The model under review builds one solid part; all positions refer to its coordinate system, in mm. Coordinates: 2 decimals unless noted, no trailing zeros. Loops run counter-clockwise (first coordinate to the right, second up) from the corner with the lowest first, then second, coordinate; pieces in that order, holes last. Notation, with made-up numbers: M 11,73.5 L 39,73.5 A21 ccw 39,92.5 Z; hole C -32,78 d6. An arc over 180 degrees is marked long. Write item = value, one per line. Start each with the question number.
Q1. We need section C-C on y = 118.25. Give the boundary of the cut face in (x, z) (1 decimal), and give its area (3 significant figures).
Q2. We need section A-A on z = -185.5. Give the boundary of the cut face in (x, y), and give its area (3 significant figures).
Q3. Wall thickness on probe 1 along Z at (x, y) = (-131, 114.5) (3 decimals); probe 2 along X at (y, z) = (118.75, -142); probe 3 along X at (y, z) = (114.5, -168): over which ranges is each line inside the solid? List them lowest first.
Q4. We need section B-B on x = -75. Give the boundary of the cut face in (y, z) (3 decimals).
Q5. Mouldability with a two-part tool opening along Z and no side actions: class faces 1 (the face through (-130.53, 116.83, -199.47)), 2 (the face through (-91, 117, -250.645)), 3 (the face through (-91, 117, -75.645)) as released by +Z, released by -Z, zero draft, split by the parting line, or undercut.
Autodesk Inventor part; units mm, degrees
ref_plane "YZ Plane" through (0, 0, 0) normal (1, 0, 0) x (0, 1, 0)
ref_plane "XZ Plane" through (0, 0, 0) normal (0, 1, 0) x (-1, 0, 0)
ref_plane "XY Plane" through (0, 0, 0) normal (0, 0, 1) x (1, 0, 0)
ref_plane "Work Plane2" through (-92.9211, 111.7581, -85.645) normal (0, 1, 0) x (-1, 0, 0)
sketch "Sketch2" plane through (-92.9211, 111.7581, -85.645) normal (0, 1, 0) x (-1, 0, 0)
  line L0 (63, 0) -> (-63, 0)
  line L1 (-63, 0) -> (-63, -150)
  line L2 (-63, -150) -> (63, -150)
  line L3 (63, -150) -> (63, 0)
  line L4 (63, 0) -> (-63, -150) construction
  line L5 (-63, 0) -> (63, -150) construction
  line L6 (-114.9576, 160) -> (114.9576, 160)
  line L7 (114.9576, 160) -> (114.9576, -160)
  line L8 (114.9576, -160) -> (-114.9576, -160)
  line L9 (-114.9576, -160) -> (-114.9576, 160)
  line L10 (119.9576, -165) -> (119.9576, 165)
  line L11 (119.9576, 165) -> (-119.9576, 165)
  line L12 (-119.9576, 165) -> (-119.9576, 10)
  line L13 (-119.9576, -165) -> (119.9576, -165)
  line L14 (-119.9576, 10) -> (-114.9576, 10)
  line L15 (-114.9576, 10) -> (114.9576, 10)
  line L16 (114.9576, 10) -> (119.9576, 10)
  line L17 (-119.9576, 10) -> (-119.9576, -165)
  point P0 (-92.9211, 85.645)
  point P1 (0, -75)
  point P2 (114.9576, 160)
  dimension "d0" = 126
  dimension "d1" = 150
  dimension "d2" = 5
  dimension "d5" = 10
  dimension "d6" = 10
extrude "Extrusion1" add sketch "Sketch2" along normal blind 10 contours L3 L2 L1 L0 | L15 L7 L8 L9 | L9 L8 L7 L16 L10 L13 L17 L14
sketch "Sketch3" plane through (-92.9211, 111.7581, -85.645) normal (0, -1, 0) x (1, 0, 0)
  line L0 (-119.9576, 10) -> (119.9576, 10)
  line L1 (-119.9576, -165) -> (-119.9576, 10)
  line L2 (119.9576, -165) -> (-119.9576, -165)
  line L3 (119.9576, 10) -> (119.9576, -165)
  line L4 (-119.9576, -165) -> (119.9576, 10)
  line L5 (-119.9576, 10) -> (119.9576, -165)
  circle A0 centre (0, -77.5) radius 37.5
  point P0 (92.9211, 85.645)
  dimension "d7" = 75
extrude "Extrusion2" cut sketch "Sketch3" against normal through all contours A0 L4 L5 | L5 L4 A0 | A0 L5 L4 | L4 L5 A0
sketch "Sketch4" plane through (-92.9211, 111.7581, -85.645) normal (0, -1, 0) x (1, 0, 0)
  circle A0 centre (-37.5, -38.6758) radius 2.5
  circle A1 centre (37.5, -38.6758) radius 2.5
  circle A2 centre (37.5, -116.3242) radius 2.5
  circle A3 centre (-37.5, -116.3242) radius 2.5
  arc A4 (47.5, -35) -> (42.5, -30) centre (42.5, -35) ccw
  line L0 (42.5, -30) -> (-42.5, -30)
  arc A5 (-42.5, -30) -> (-47.5, -35) centre (-42.5, -35) ccw
  line L1 (-47.5, -35) -> (-47.5, -120)
  arc A6 (-47.5, -120) -> (-42.5, -125) centre (-42.5, -120) ccw
  line L2 (-42.5, -125) -> (42.5, -125)
  arc A7 (42.5, -125) -> (47.5, -120) centre (42.5, -120) ccw
  line L3 (47.5, -120) -> (47.5, -35)
  circle A8 centre (0, -77.5) radius 5
  point P0 (92.9211, 85.645)
hole "Hole1" at (-130.4211, 111.7581, -124.3208) at (-55.4211, 111.7581, -124.3208) at (-55.4211, 111.7581, -201.9692) at (-130.4211, 111.7581, -201.9692) direction (0, 1, 0) diameter 5 end through all
properties part number "Sleed_Plate"
Returned:
q1.outline = M -212.9,-250.6 L 27,-250.6 L 27,-75.6 L -212.9,-75.6 Z; hole C -130.4,-202 d5; hole C -130.4,-124.3 d5; hole C -92.9,-163.1 d75; hole C -55.4,-202 d5; hole C -55.4,-124.3 d5
q1.area = 37,500 mm^2
q2.outline = M -212.88,111.76 L -123.03,111.76 L -123.03,121.76 L -212.88,121.76 Z; M -62.81,111.76 L 27.04,111.76 L 27.04,121.76 L -62.81,121.76 Z
q2.area = 1,800 mm^2
q3.probe_1 = -250.645 to -204.401, -199.537 to -126.753, -121.889 to -75.645
q3.probe_2 = -212.88 to -123.89, -61.95 to 27.04
q3.probe_3 = -212.88 to -130.11, -55.74 to 27.04
q4.outline = M 111.758,-250.645 L 121.758,-250.645 L 121.758,-196.086 L 111.758,-196.086 Z; M 111.758,-130.204 L 121.758,-130.204 L 121.758,-75.645 L 111.758,-75.645 Z
q5.face_1 = undercut
q5.face_2 = released by -Z
q5.face_3 = released by +Z
